Can you work these out from the model? Positions are in its coordinate system, mm. A direction names the side the tool comes from. Round coordinates to 2 decimals unless told otherwise and drop trailing zeros. Loops run counter-clockwise (first coordinate to the right, second up) from the corner with the lowest first, then second, coordinate; pieces in that order, holes last.
(1) If I drill on line 1 along Y through (x, z) = (0, 3.6); line 2 along X through (y, z) = (13.5, 2.75); line 3 along Y through (x, z) = (-1, 0.75), over which ranges is the centre line in solid material (lowest first)?
(2) I want a section at B-B on z = 12. Write out the boundary of the cut face in (x, y), plus the area to 3 significant figures.
(3) Thinking about a two-plate mould opening in X: for faces 1 (the face through (0, -17, 3)), 2 (the face through (-2.247, 0, 7)), 3 (the face through (23.846, 7.509, 2.47)), 4 (the face through (11, -11, 5)), which applies, released by +X, released by -X, zero draft, split by the parting line, or undercut?
(4) Which directions (+Z, -Z, +X, -X, +Y, -Y) give clear straight access to the entire face, cutting with the end or side of a thin tool? Please do faces 5 (the face through (-10.316, -7.91, 9.753)), 6 (the face through (0, 21, 3)).
(5) Will these pins go through, and if not, where does the flat tip stop? pin 1 Ø3 at (x, y) = (0, -19) entering from -Z; pin 2 Ø5 at (x, z) = (-14, 11.5) entering from -Y; pin 3 Ø2 at (y, z) = (-5.5, 12.5) entering from -X; pin 4 Ø8 at (x, y) = (-13.5, 13.5) entering from +Z.
(6) I want a section at A-A on x = 0. Write out the boundary of the cut face in (y, z), plus the area to 3 significant figures.
from build123d import *

# Parameters (mm, degrees)
SKETCH_1_R          = 25
SKETCH_1_R_2        = 4
EXTRUDE_1_DEPTH     = 5
EXTRUDE_2_DEPTH     = 5
SKETCH_5_R          = 13
EXTRUDE_3_DEPTH     = 10
CUT_EXTRUDE_1_DEPTH = 18
SKETCH_7_R          = 2
CUT_EXTRUDE_2_DEPTH = 18
FILLET_4_R          = 0.36


with BuildPart() as part:
    # 草图1 → 凸台-拉伸1 (new body)
    with BuildSketch(Plane.XY):
        Circle(SKETCH_1_R)
        Circle(SKETCH_1_R_2, mode=Mode.SUBTRACT)
    extrude(amount=EXTRUDE_1_DEPTH)

    # 草图2 → 凸台-拉伸2 (add)
    with BuildSketch(Plane.XY.offset(5)):
        with BuildLine():
            Line((-2.247476495, -3.308904563), (-2.247476495, 3.308904563))
            ThreePointArc((-2.247476495, 3.308904563), (-4, 0), (-2.247476495, -3.308904563))
        make_face()
    extrude(amount=-EXTRUDE_2_DEPTH)

    # 草图5 → 凸台-拉伸3 (add)
    with BuildSketch(Plane.XY.offset(5)):
        Circle(SKETCH_5_R)
    extrude(amount=EXTRUDE_3_DEPTH)

    # 草图6 → 切除-拉伸1 (cut)
    with BuildSketch(Plane(origin=(0, 0, 0), x_dir=(-1, 0, 0), z_dir=(0, 0, -1))):
        with BuildLine():
            Line((2.247476495, 3.308904563), (2.247476495, -3.308904563))
            ThreePointArc((2.247476495, -3.308904563), (-4, 0), (2.247476495, 3.308904563))
        make_face()
    extrude(amount=-CUT_EXTRUDE_1_DEPTH, mode=Mode.SUBTRACT)

    # 草图7 → 切除-拉伸2 (cut)
    with BuildSketch(Plane.XY.offset(5)):
        with Locations((0, 19)):
            Circle(SKETCH_7_R)
        with Locations((13.435028843, 13.435028843)):
            Circle(SKETCH_7_R)
        with Locations((19, 0)):
            Circle(SKETCH_7_R)
        with Locations((13.435028843, -13.435028843)):
            Circle(SKETCH_7_R)
        with Locations((0, -19)):
            Circle(SKETCH_7_R)
        with Locations((-13.435028843, -13.435028843)):
            Circle(SKETCH_7_R)
        with Locations((-19, 0)):
            Circle(SKETCH_7_R)
        with Locations((-13.435028843, 13.435028843)):
            Circle(SKETCH_7_R)
    extrude(amount=-CUT_EXTRUDE_2_DEPTH, mode=Mode.SUBTRACT)

    # 圆角4
    fillet_4_edges = [part.edges().sort_by_distance(p)[0] for p in [
        (-25, 0, 0),
        (-13, 0, 15),
        (-25, 0, 5),
    ]]
    fillet(fillet_4_edges, radius=FILLET_4_R)


solid = part.part
Filled sheet:
1. line 1: y = -25 to -21, -17 to -4, 4 to 17, 21 to 25
1. line 2: x = -21.04 to -15.43, -11.44 to 11.44, 15.43 to 21.04
1. line 3: y = -24.98 to -20.73, -17.27 to -3.87, 3.87 to 17.27, 20.73 to 24.98
2. outline: circle Ø26 at (0, 0); hole (-2.25, -3.31) arc R4 ccw (long way) to (-2.25, 3.31) - close
2. area: 489 mm2
3. face 1: undercut
3. face 2: undercut
3. face 3: split by the parting line
3. face 4: zero draft
4. face 5: +Z
4. face 6: +Z, -Z
5. pin 1: passes through
5. pin 2: stops at y = -6.06
5. pin 3: stops at x = -12.2
5. pin 4: stops at z = 5
6. outline: (-25, 0.36) arc R0.36 ccw to (-24.64, 0) - (-21, 0) - (-21, 5) - (-24.64, 5) arc R0.36 ccw to (-25, 4.64) - close; (-17, 0) - (-4, 0) - (-4, 15) - (-12.64, 15) arc R0.36 ccw to (-13, 14.64) - (-13, 5) - (-17, 5) - close; (4, 0) - (17, 0) - (17, 5) - (13, 5) - (13, 14.64) arc R0.36 ccw to (12.64, 15) - (4, 15) - close; (21, 0) - (24.64, 0) arc R0.36 ccw to (25, 0.36) - (25, 4.64) arc R0.36 ccw to (24.64, 5) - (21, 5) - close
6. area: 350 mm2
